from build123d import *

# Parameters (mm, degrees)
F0_W     = 58.9215288217
F0_H     = 8.9712000314
F0_H_2   = 1.1887999686
F0_W_2   = 50.8
F0_H_3   = 93.8377175136
F0_H_4   = 50.346628223
F0_H_5   = 109.2197667617
F0_H_6   = 30.6704640388
F1_DEPTH = 38.1


with BuildPart() as f1:
    # F0 (on Front) → F1 (new body, symmetric)
    with BuildSketch(Plane.XZ):
        Polygon((-52.8541674206, 65.5549615622), (-52.8541674206, -9.8338549508), (-30.4587072518, -9.8338549508), (28.4628215698, -9.8338549508), (48.7458325794, -9.8338549508), (48.7458325794, 71.4190080762), (33.4042608738, 71.4190080762), (33.4042608738, 75.9503096342), (8.8818948716, 75.9503096342), (8.8818948716, 71.6855600476), (-20.7048710436, 71.6855600476), (-20.7048710436, 79.6819776297), (-47.3596155643, 79.6819776297), (-47.3596155643, 65.5549615622), align=None)
        Polygon((-18.5442172647, 45.2312529087), (-43.9442172647, 45.2312529087), (-43.9442172647, 70.6312529087), (-31.2442172647, 70.6312529087), (-18.5442172647, 70.6312529087), (-18.5442172647, 53.8268759847), align=None, mode=Mode.SUBTRACT)
        Polygon((43.9442172647, 45.2312529087), (18.5442172647, 45.2312529087), (18.5442172647, 70.6312529087), (31.2442172647, 70.6312529087), (43.9442172647, 70.6312529087), (43.9442172647, 53.8268759847), align=None, mode=Mode.SUBTRACT)
        with Locations((-0.997942841, -14.3194549665)):
            Rectangle(F0_W, F0_H)
        Polygon((-52.8541674206, 91.7661450492), (-52.8541674206, 65.5549615622), (-47.3596155643, 65.5549615622), (-47.3596155643, 79.6819776297), (-20.7048710436, 79.6819776297), (-20.7048710436, 71.6855600476), (8.8818948716, 71.6855600476), (8.8818948716, 75.9503096342), (33.4042608738, 75.9503096342), (33.4042608738, 71.4190080762), (48.7458325794, 71.4190080762), (48.7458325794, 91.7661450492), align=None)
        with Locations((-0.997942841, -19.3994549665)):
            Rectangle(F0_W, F0_H_2)
        Polygon((-30.4587072518, -19.9938549508), (-30.4587072518, -18.8050549821), (-50.8, -18.8050549821), (-50.8, -112.6427724957), (-50.8, -162.9894007187), (0, -162.9894007187), (50.8, -162.9894007187), (50.8, -112.6427724957), (50.8, -18.8050549821), (28.4628215698, -18.8050549821), (28.4628215698, -19.9938549508), align=None)
        with Locations((-76.2, -65.7239137389)):
            Rectangle(F0_W_2, F0_H_3)
        Polygon((53.1537466286, -18.8050549821), (50.8, -18.8050549821), (50.8, -112.6427724957), (101.6, -112.6427724957), (101.6, -18.8050549821), align=None)
        with Locations((-76.2, -137.8160866072)):
            Rectangle(F0_W_2, F0_H_4)
        with Locations((76.2, -137.8160866072)):
            Rectangle(F0_W_2, F0_H_4)
        with Locations((-25.4, -217.5992840996)):
            Rectangle(F0_W_2, F0_H_5)
        with Locations((25.4, -217.5992840996)):
            Rectangle(F0_W_2, F0_H_5)
        with Locations((-25.4, -287.5443994999)):
            Rectangle(F0_W_2, F0_H_6)
        with Locations((25.4, -287.5443994999)):
            Rectangle(F0_W_2, F0_H_6)
    extrude(amount=F1_DEPTH, both=True)


solid = f1.part
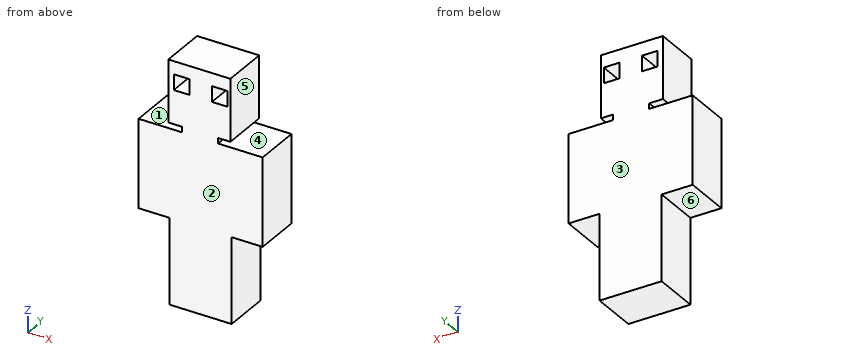
Here's how the part is built. I have some questions about the finished solid (model axes, mm). Face numbers are marked on the shaded views. A direction names the side the tool comes from. Round coordinates to 2 decimals unless told otherwise and drop trailing zeros. Order: outer loops, then holes, each group sorted by start corner. A loop starts at its lowest first (then second) coordinate and runs counter-clockwise, first axis right, second up. Notation, with made-up numbers: (-39, -5.5) -> (-23, -5.5) arc R35 ccw to (-23, 26.5) -> close; hole circle Ø7 at (26, 19.5). An arc over 180 degrees is marked (long way). Use CSV: the item, a comma, the result in double quotes.
1. I want a section at D-D on z = -195. List the corners of the cut face in (x, y) for me, and give its area (3 significant figures).
Recorded:
outline,"(-50.8, -38.1) -> (50.8, -38.1) -> (50.8, 38.1) -> (-50.8, 38.1) -> close"
area,"7,740 mm2"
2. Thinking about a two-plate mould opening in Y: for the marked faces 1, 2 and 3, which applies, pulls with the +Y half, pulls with the -Y half, needs draft (parallel to the pull), parting line crosses it, or undercut?
Recorded:
face 1,"needs draft"
face 2,"pulls with the -Y half"
face 3,"pulls with the +Y half"
3. I want a section at C-C on x = -87. List the corners of the cut face in (y, z) for me, and give its area (3 significant figures).
Recorded:
outline,"(-38.1, -162.99) -> (38.1, -162.99) -> (38.1, -18.81) -> (-38.1, -18.81) -> close"
area,"11,000 mm2"
4. I'm going to push flat-ended pins straight in: P1, Ø10, axis at y = 13, z = -260.5, coming from the +X side; P2, Ø23, axis at y = -9.5, z = -243, coming from the -X side; P3, Ø12.5, axis at y = -8, z = 59.5, coming from the -X side. Where does each tip first touch, or does it pass through?
Recorded:
P1,"stops at x = 50.8"
P2,"stops at x = -50.8"
P3,"stops at x = -52.85"
5. Which directions (+Z, -Z, +X, -X, +Y, -Y) give clear straight access to the entire face, cutting with the end or side of a thin tool? Please do the marked faces 4, 5 and 6.
Recorded:
face 4,"+X, +Y, -Y"
face 5,"+Z, +X, +Y, -Y"
face 6,"-Z, -X, +Y, -Y"
6. I want a section at B-B on y = -22. List the corners of the cut face in (x, z) for me.
Recorded:
outline,"(-101.6, -162.99) -> (-50.8, -162.99) -> (-50.8, -302.88) -> (50.8, -302.88) -> (50.8, -162.99) -> (101.6, -162.99) -> (101.6, -18.81) -> (28.46, -18.81) -> (28.46, -9.83) -> (48.75, -9.83) -> (48.75, 91.77) -> (-52.85, 91.77) -> (-52.85, -9.83) -> (-30.46, -9.83) -> (-30.46, -18.81) -> (-101.6, -18.81) -> close; hole (-43.94, 45.23) -> (-18.54, 45.23) -> (-18.54, 70.63) -> (-43.94, 70.63) -> close; hole (18.54, 45.23) -> (43.94, 45.23) -> (43.94, 70.63) -> (18.54, 70.63) -> close"
7. I need wall thicknesses on line 1 along Z through (x, y) = (38.5, -29); line 2 along Z through (x, y) = (-25, 31.5); line 3 along X through (y, z) = (-12.5, -257). Which ranges of each line are inside material? Lowest first, please.
Recorded:
line 1,"z = -302.88 to -18.81, -9.83 to 45.23, 70.63 to 91.77"
line 2,"z = -302.88 to 45.23, 70.63 to 91.77"
line 3,"x = -50.8 to 50.8"
8. I want a section at A-A on x = -23.5. List the corners of the cut face in (y, z) for me, and give its area (3 significant figures).
Recorded:
outline,"(-38.1, -302.88) -> (38.1, -302.88) -> (38.1, 45.23) -> (-38.1, 45.23) -> close; (-38.1, 70.63) -> (38.1, 70.63) -> (38.1, 91.77) -> (-38.1, 91.77) -> close"
area,"28,100 mm2"
